from build123d import *

# Parameters (mm, degrees)
F0_W     = 37
F0_H     = 24
F0_R     = 0.3
F1_DEPTH = 15
F2_DEPTH = 18.5
F3_ANGLE = 180


with BuildPart() as f1:
    # F0 (on Top) → F1 (new body)
    with BuildSketch(Plane.XY):
        Rectangle(F0_W, F0_H)
        with Locations((10.16, -8.89)):
            Circle(F0_R, mode=Mode.SUBTRACT)
        with Locations((15.24, -8.89)):
            Circle(F0_R, mode=Mode.SUBTRACT)
        with Locations((-15.24, 8.89)):
            Circle(F0_R, mode=Mode.SUBTRACT)
        with Locations((-10.16, 8.89)):
            Circle(F0_R, mode=Mode.SUBTRACT)
        with Locations((15.24, 8.89)):
            Circle(F0_R, mode=Mode.SUBTRACT)
    extrude(amount=F1_DEPTH)

    # F0 (on Top) → F2 (join)
    with BuildSketch(Plane.XY):
        with Locations((15.24, 8.89)):
            Circle(F0_R)
        with Locations((-10.16, 8.89)):
            Circle(F0_R)
        with Locations((-15.24, 8.89)):
            Circle(F0_R)
        with Locations((15.24, -8.89)):
            Circle(F0_R)
        with Locations((10.16, -8.89)):
            Circle(F0_R)
    extrude(amount=F2_DEPTH)


with BuildPart() as f1_1:
    # F3: moved
    add(f1.part.rotate(Axis((0, -12, 15), (1, 0, 0)), F3_ANGLE))


solid = f1_1.part
Can you work these out from the model? Positions are in its coordinate system, mm. Give positions to 0.01 mm unless a question says otherwise; leave off trailing zeros. Loops run counter-clockwise (first coordinate to the right, second up) from the corner with the lowest first, then second, coordinate; pieces in that order, holes last. Notation, with made-up numbers: (-17, 17.5) - (-2, 17.5) arc R30 cw to (-2, 51.5) - close; hole circle Ø11 at (-7, -27). An arc over 180 degrees is marked (long way). Answer as a JSON object with one key per item and string values.
Q1. If I drill on L1, parallel to Z at x = 8, y = -22; L2, parallel to Y at x = 15, z = 14.75, over which ranges is the centre line in solid material (lowest first)?
Geometry says:
{"L1": "15 to 30", "L2": "-33.07 to -32.71, -15.29 to -14.93"}
Q2. Will this pin go through, and if not, where does the flat tip stop? P1, Ø3, axis at x = 12, y = -21.5, coming from the -Z side.
Geometry says:
{"P1": "z = 15"}
Q3. Imagine slicing it at A-A on y = -14. Write out the boundary of the cut face in (x, z), plus the area to 3 significant figures.
Geometry says:
{"outline": "(-18.5, 15) - (18.5, 15) - (18.5, 30) - (-18.5, 30) - close", "area": "555 mm²"}
Q4. Imagine slicing it at B-B on x = -2.5. Write out the boundary of the cut face in (y, z).
Geometry says:
{"outline": "(-36, 15) - (-12, 15) - (-12, 30) - (-36, 30) - close"}
